from build123d import *

# Parameters (mm, degrees)
SKETCH1_W             = 43.18
SKETCH1_H             = 43.18
BOSS_EXTRUDE1_DEPTH   = 15
M3X0_5_TAPPED_HOLE1_D = 2.5
CHAMFER1_SIZE         = 0.5


with BuildPart() as part:
    # Sketch1 → Boss-Extrude1 (new body)
    with BuildSketch(Plane(origin=(0, 0, 0), x_dir=(1, 0, 0), z_dir=(0, 1, 0))):
        Rectangle(SKETCH1_W, SKETCH1_H)
    extrude(amount=BOSS_EXTRUDE1_DEPTH)

    # M3x0.5 Tapped Hole1 (through all)
    with Locations(Plane(origin=(0, 15, 0), x_dir=(1, 0, 0), z_dir=(0, 1, 0))):
        with Locations((-18.669, -17.272), (-9.144, 18.923), (18.161, 0.762)):
            Hole(M3X0_5_TAPPED_HOLE1_D / 2)

    # Chamfer1
    chamfer1_edges = [part.edges().sort_by_distance(p)[0] for p in [
        (21.59, 0, 0),
        (0, 0, 21.59),
        (-21.59, 0, 0),
        (0, 0, -21.59),
    ]]
    chamfer(chamfer1_edges, length=CHAMFER1_SIZE)


solid = part.part
Verification items for the finished model (mm, model axes). Give positions to 0.01 mm unless a question says otherwise; leave off trailing zeros. Order: outer loops, then holes, each group sorted by start corner. A loop starts at its lowest first (then second) coordinate and runs counter-clockwise, first axis right, second up. Notation, with made-up numbers: M 36.25,42.25 L 41.25,42.25 A27 cw 41.25,77.25 Z; hole C 8.25,36.25 d3. An arc over 180 degrees is marked long. Use one line per item in the form item = value. Start each with the question number.
Q1. Section check A-A (x = -8.5). Enter the section's corners in (y, z), then the cut area to 3 significant figures.
Q2. Mould release check, pull along X, two halves, no side actions. Record for faces 1 (the flat face through (21.59, 8, 0)), 2 (the flat face through (0, 8, 21.59)), 3 (the cylindrical face through (-7.895, 7.395, -18.978)): +X half, -X half, draft (parallel to the pull), parting line (faces both ways), or undercut.
Q3. Scan lines: line 1 along Z through (x, y) = (-9, 12.25); line 2 along Z through (x, y) = (-9.5, 3.5); line 3 along X through (y, z) = (9.75, -1). Record each from-to range of solid material in increasing order. Write a range as [from, to].
Evaluation:
q1.outline = M 0,-21.09 L 0.5,-21.59 L 15,-21.59 L 15,-19.99 L 0,-19.99 Z; M 0,-17.85 L 15,-17.85 L 15,21.59 L 0.5,21.59 L 0,21.09 Z
q1.area = 615 mm2
q2.face_1 = +X half
q2.face_2 = draft
q2.face_3 = undercut
q3.line_1 = [-21.59, -20.16], [-17.68, 21.59]
q3.line_2 = [-21.59, -20.12], [-17.72, 21.59]
q3.line_3 = [-21.59, 16.93], [19.39, 21.59]
